The listing builds one solid part. Answer for the finished solid, in the listing's coordinates (mm). A direction names the side the tool comes from. Round coordinates to 2 decimals unless told otherwise and drop trailing zeros. Write each loop counter-clockwise with the first axis right and the second up, starting at its lowest first coordinate (ties: lowest second). Pieces come first, ordered by that corner, then holes.
(1) A cutting plane is placed at A-A, the plane z = -2. Give the vertices of the cut face in (x, y), and give its area (3 significant figures).
(2) Each of these flat-tipped pins is pushed along its axis until it touches: pin 1 Ø4 at (x, y) = (-14.5, 14) entering from +Z; pin 2 Ø2 at (x, z) = (-4.5, -6.5) entering from -Y; pin 3 Ø6 at (x, z) = (-13.5, -15.5) entering from +Y; pin 4 Ø2.5 at (x, z) = (-12.5, 3) entering from +Y. Where does it stop, or does it pass through?
(3) Find the intervals of material crossed by probe 1 along Y at (x, z) = (-11, 2); probe 2 along Z at (x, y) = (-6, 12.5); probe 3 along Y at (x, z) = (-5, -16.5), in increasing order.
(4) For faces 1 (the face through (-10, 1, 2)), 2 (the face through (-18, 48, -33)), 3 (the face through (-2.8, 47, -2.6)), determine the directions among +Z, -Z, +X, -X, +Y, -Y from which every point of the face is accessible in a straight line to the end or side of a thin tool.
(5) The mould has two halves that part along X. Classify faces 4 (the face through (-20, 23, -19)), 5 (the face through (-18, 47, -32)), 6 (the face through (-18, 48, -2)): +X half, -X half, draft (parallel to the pull), parting line (faces both ways), or undercut.
(6) A cutting plane is placed at C-C, the plane y = 25.5. Give the vertices of the cut face in (x, z).
(7) A cutting plane is placed at B-B, the plane x = -4. Give the vertices of the cut face in (y, z).
Autodesk Inventor part; units mm, degrees
ref_plane "YZ Plane" through (0, 0, 0) normal (1, 0, 0) x (0, 1, 0)
ref_plane "XZ Plane" through (0, 0, 0) normal (0, 1, 0) x (-1, 0, 0)
ref_plane "XY Plane" through (0, 0, 0) normal (0, 0, 1) x (1, 0, 0)
sketch "Sketch1" plane through (0, 0, 0) normal (0, 1, 0) x (-1, 0, 0)
  line L0 (0, 0) -> (20, 0)
  line L1 (20, 0) -> (20, -35)
  line L2 (20, -35) -> (0, -35)
  line L3 (0, -35) -> (0, 0)
  dimension "d0" = 20
  dimension "d1" = 35
extrude "Extrusion1" add sketch "Sketch1" along normal blind 46
sketch "Sketch2" plane through (-20, 0, 0) normal (0, 0, 1) x (1, 0, 0)
  line L0 (0, 0) -> (0, 46)
  line L1 (20, 0) -> (20, 46)
  line L2 (0, 0) -> (20, 0)
  line L3 (20, 0) -> (20, 1)
  line L4 (20, 1) -> (0, 1)
  line L5 (0, 1) -> (0, 0)
  dimension "d4" = 1
extrude "Extrusion2" add sketch "Sketch2" along normal blind 6
sketch "Sketch3" plane through (-20, 1, 0) normal (0, 1, 0) x (1, 0, 0)
  line L0 (0, 35) -> (0, -6)
  line L1 (20, 35) -> (20, -6)
  line L2 (0, -6) -> (20, -6)
  line L3 (20, -6) -> (20, -5)
  line L4 (20, -5) -> (0, -5)
  line L5 (0, -5) -> (0, -6)
  point P0 (20, 0)
  dimension "d7" = 1
extrude "Extrusion3" add sketch "Sketch3" along normal blind 5
fillet "Fillet1" radius 2 1 edges at (-10, 6, 6)
sketch "Sketch4" plane through (0, 46, 0) normal (0, 1, 0) x (1, 0, 0)
  arc A0 (-20, 2) -> (-18, 0) centre (-18, 2) ccw
  circle A1 centre (-18, 2) radius 1
  arc A2 (-2, 0) -> (0, 2) centre (-2, 2) ccw
  circle A3 centre (-2, 2) radius 1
  arc A4 (0, 33) -> (-2, 35) centre (-2, 33) ccw
  circle A5 centre (-2, 33) radius 1
  arc A6 (-18, 35) -> (-20, 33) centre (-18, 33) ccw
  circle A7 centre (-18, 33) radius 1
  point P0 (0, 0)
  dimension "d11" = 2
  dimension "d12" = 2
  dimension "d13" = 2
  dimension "d14" = 2
extrude "Extrusion4" add sketch "Sketch4" along normal blind 2
properties part number "platform"
Solutions:
1. outline: (-20, 0) - (0, 0) - (0, 46) - (-1, 46) - (-1, 48) - (-3, 48) - (-3, 46) - (-17, 46) - (-17, 48) - (-19, 48) - (-19, 46) - (-20, 46) - close
1. area: 928 mm2
2. pin 1: stops at z = 0
2. pin 2: stops at y = 0
2. pin 3: stops at y = 46
2. pin 4: stops at y = 1
3. probe 1: y = 0 to 1
3. probe 2: z = -35 to 0
3. probe 3: y = 0 to 46
4. face 1: +X, -X, +Y
4. face 2: +Z, -Z, +X, -X, +Y
4. face 3: +Y
5. face 4: -X half
5. face 5: undercut
5. face 6: draft
6. outline: (-20, -35) - (0, -35) - (0, 0) - (-20, 0) - close
7. outline: (0, -35) - (46, -35) - (46, 0) - (1, 0) - (1, 5) - (6, 5) arc R2 ccw to (4.27, 6) - (0, 6) - close
